CAD build for the part. Positions are in the model's coordinates, mm. Face numbers are marked on the shaded views. A direction names the side the tool comes from. Give positions to 0.01 mm unless a question says otherwise; leave off trailing zeros. Write each loop counter-clockwise with the first axis right and the second up, starting at its lowest first coordinate (ties: lowest second). Pieces come first, ordered by that corner, then holes. Notation, with made-up numbers: M 5.5,-5 L 42.5,-5 A36 cw 42.5,34 Z; hole C -9.75,2.5 d7. An arc over 180 degrees is marked long. One line per question, with ' | ' between items. Start each with the question number.
1. Pull direction Y, two halves, no side cores. Call the marked faces 4, 5, 6 and 7: released by +Y, released by -Y, zero draft, split by the parting line, or undercut.
2. Wall check: L1, parallel to X at y = 37.5, z = -5; L2, parallel to X at y = 42, z = 4.25; L3, parallel to Y at x = -43, z = 4. Give the ranges that are in metal, low to high.
3. Flat gauge pins, fed straight in: pin 1 (0.7 mm diameter, centred on y = 20.5, z = -6, fed in from +X); pin 2 (2 mm diameter, centred on y = 32, z = -1, fed in from -X). Where does each tip first touch, or does it go through?
4. Cut at A-A, the plane z = -4. Write the cut outline in (x, y), then the cut area to 3 significant figures.
5. Which spindle directions (+Z, -Z, +X, -X, +Y, -Y) get a long thin tool onto all of the face, cutting with end or side? Do the marked faces 1, 2 and 3. Say none if no direction does.
```python
from build123d import *

# Parameters (mm, degrees)
F3_DEPTH = 6.35
F4_DEPTH = 5.715


with BuildPart() as f3:
    # F2 (on face) → F3 (new body, symmetric)
    with BuildSketch(Plane.XY):
        Polygon((-44.5433743298, 46.1763069034), (-57.5266592205, 46.1332164705), (-57.5266592205, 35.8126908541), (-54.5913651586, 35.8126908541), (-54.5913651586, 14.4700501114), (-57.5266592205, 14.4700501114), (-57.5266592205, 4.1293082759), (-41.6378863156, 4.1293082759), (-41.6378863156, 14.4700501114), (-44.5433743298, 14.4700501114), (-44.5433743298, 28.3214543015), (-29.1992705315, 4.1293082759), (-15.6220048666, 4.1293082759), (-15.6220048666, 14.4700501114), (-18.5752976686, 14.4700501114), (-18.5752976686, 35.8126908541), (-15.6220048666, 35.8126908541), (-15.6220048666, 46.1763069034), (-31.5383896232, 46.1763069034), (-31.5383896232, 35.8126908541), (-28.6253094673, 35.8126908541), (-28.6253094673, 21.92475833), align=None)
    extrude(amount=F3_DEPTH, both=True)



with BuildPart() as f3b:
    # F1 (on face) → F3, piece 2 (new body, symmetric)
    with BuildSketch(Plane.XY):
        Polygon((-56.0555362153, 34.3240606943), (-56.0555362153, 15.9201806872), (-59.0018344771, 15.9201806872), (-59.0018344771, 2.6492023655), (-40.1264553645, 2.6492023655), (-40.1264553645, 15.9219650984), (-43.0878697398, 15.9219650984), (-43.0878697398, 23.2951258444), (-30.0034182126, 2.6492023655), (-14.1497837651, 2.6492023655), (-14.1497837651, 15.9219650984), (-17.0993286024, 15.9219650984), (-17.0993286024, 34.3240606943), (-14.1497837651, 34.3240606943), (-14.1497837651, 47.5996589474), (-33.0122411207, 47.5996589474), (-33.0122411207, 34.3240606943), (-30.0034182126, 34.3240606943), (-30.0034182126, 26.9455498071), (-43.0878697398, 47.5996589474), (-59.0018344771, 47.5996589474), (-59.0018344771, 34.3240606943), align=None)
        Polygon((-58.4264323115, 34.9163971841), (-58.4264323115, 46.9940491021), (-43.5850694776, 47.013964504), (-29.5001640916, 24.9555353075), (-29.5001640916, 34.9163971841), (-32.4371978641, 34.9163971841), (-32.4371978641, 47.013964504), (-14.7387757897, 47.013964504), (-14.7387757897, 34.9163971841), (-17.6595617086, 34.9163971841), (-17.6595617086, 15.3841460124), (-14.7387757897, 15.3841460124), (-14.7387757897, 3.2841966022), (-29.7212973237, 3.2841966022), (-43.5850694776, 25.176089257), (-43.5850694776, 15.3841460124), (-40.7384447753, 15.3841460124), (-40.7384447753, 3.2841966022), (-58.4264323115, 3.2841966022), (-58.4264323115, 15.3841460124), (-55.4955154657, 15.3841460124), (-55.4955154657, 34.9163971841), align=None, mode=Mode.SUBTRACT)
    extrude(amount=F3_DEPTH, both=True)


with BuildPart() as f3_1:
    add(f3.part)

    add(f3b.part)  # F4 merges F3b
    # F2 (on face) → F4 (join, symmetric)
    with BuildSketch(Plane.XY):
        Polygon((-58.4264323115, 46.9940491021), (-58.4264323115, 34.9163971841), (-55.4955154657, 34.9163971841), (-55.4955154657, 15.3841460124), (-58.4264323115, 15.3841460124), (-58.4264323115, 3.2841966022), (-40.7384447753, 3.2841966022), (-40.7384447753, 15.3841460124), (-43.5850694776, 15.3841460124), (-43.5850694776, 25.176089257), (-29.7212973237, 3.2841966022), (-14.7387757897, 3.2841966022), (-14.7387757897, 15.3841460124), (-17.6595617086, 15.3841460124), (-17.6595617086, 34.9163971841), (-14.7387757897, 34.9163971841), (-14.7387757897, 47.013964504), (-32.4371978641, 47.013964504), (-32.4371978641, 34.9163971841), (-29.5001640916, 34.9163971841), (-29.5001640916, 24.9555353075), (-43.5850694776, 47.013964504), align=None)
        Polygon((-57.5266592205, 35.8126908541), (-57.5266592205, 46.1332164705), (-44.5433743298, 46.1763069034), (-28.6253094673, 21.92475833), (-28.6253094673, 35.8126908541), (-31.5383896232, 35.8126908541), (-31.5383896232, 46.1763069034), (-15.6220048666, 46.1763069034), (-15.6220048666, 35.8126908541), (-18.5752976686, 35.8126908541), (-18.5752976686, 14.4700501114), (-15.6220048666, 14.4700501114), (-15.6220048666, 4.1293082759), (-29.1992705315, 4.1293082759), (-44.5433743298, 28.3214543015), (-44.5433743298, 14.4700501114), (-41.6378863156, 14.4700501114), (-41.6378863156, 4.1293082759), (-57.5266592205, 4.1293082759), (-57.5266592205, 14.4700501114), (-54.5913651586, 14.4700501114), (-54.5913651586, 35.8126908541), align=None, mode=Mode.SUBTRACT)
    extrude(amount=F4_DEPTH, both=True)


solid = f3_1.part
```
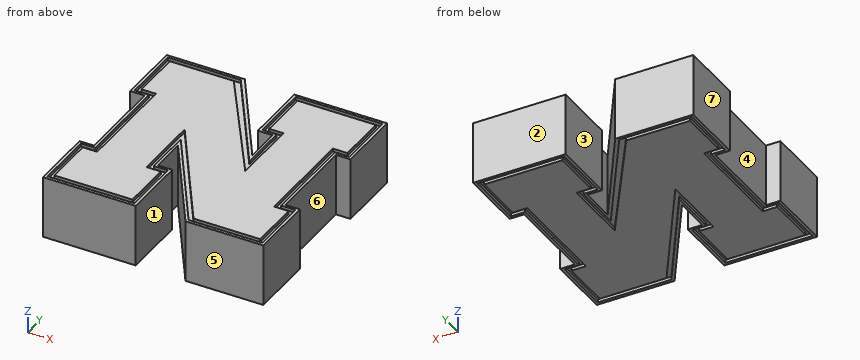
Here are the results:
1) face 4: undercut | face 5: released by -Y | face 6: undercut | face 7: zero draft
2) L1: -59 to -36.69, -33.01 to -14.15 | L2: -59 to -39.54, -33.01 to -14.15 | L3: 2.65 to 15.92, 23.16 to 47.46
3) pin 1: x = -17.1 | pin 2: x = -56.06
4) outline: M -59,2.65 L -40.13,2.65 L -40.13,15.92 L -43.09,15.92 L -43.09,23.3 L -30,2.65 L -14.15,2.65 L -14.15,15.92 L -17.1,15.92 L -17.1,34.32 L -14.15,34.32 L -14.15,47.6 L -33.01,47.6 L -33.01,34.32 L -30,34.32 L -30,26.95 L -43.09,47.6 L -59,47.6 L -59,34.32 L -56.06,34.32 L -56.06,15.92 L -59,15.92 Z | area: 1,720 mm^2
5) face 1: +Z, -Z, -Y | face 2: +Z, -Z, +X, -X, +Y | face 3: +Z, -Z, +Y
